from build123d import *

# Parameters (mm, degrees)
CUT_EXTRUDE1_DEPTH = 16.684387141
CIRPATTERN1_COUNT  = 6


with BuildPart() as part:
    # Sketch1 → Revolve1 (revolve)
    with BuildSketch(Plane.XY, mode=Mode.PRIVATE) as revolve1_sk:
        with BuildLine():
            Line((-5, 9), (-1.125, 9))
            Line((-1.125, 9), (-1.125, 4))
            Line((-1.125, 4), (0, 4))
            Line((0, 4), (0, -5))
            ThreePointArc((0, -5), (-3.535533906, -3.535533906), (-5, 0))
            Line((-5, 0), (-5, 9))
        make_face()
    revolve(revolve1_sk.sketch.rotate(Axis((0, 0, 0), (0, 1, 0)), 270), axis=Axis((0, 0, 0), (0, 1, 0)))

    # Sketch2 → Cut-Extrude1 (cut, through all)
    with BuildSketch(Plane(origin=(0, 9, 0), x_dir=(1, 0, 0), z_dir=(0, 1, 0))):
        with BuildLine():
            Line((-4.94979148, -0.706798632), (-3.36819132, 0))
            ThreePointArc((-3.36819132, 0), (-3.260778077, 0.247971643), (-3.498444432, 0.376588299))
            Line((-3.498444432, 0.376588299), (-5, 0))
            ThreePointArc((-5, 0), (-4.987432075, -0.354289854), (-4.94979148, -0.706798632))
        make_face()
    cut_extrude1 = extrude(amount=-CUT_EXTRUDE1_DEPTH, mode=Mode.SUBTRACT)

    # CirPattern1: Cut-Extrude1 ×6 about axis
    cirpattern1_axis = Axis((0, 0, 0), (0, 1, 0))
    for i in range(1, CIRPATTERN1_COUNT):
        add(cut_extrude1.rotate(cirpattern1_axis, i * 360 / CIRPATTERN1_COUNT), mode=Mode.SUBTRACT)


solid = part.part
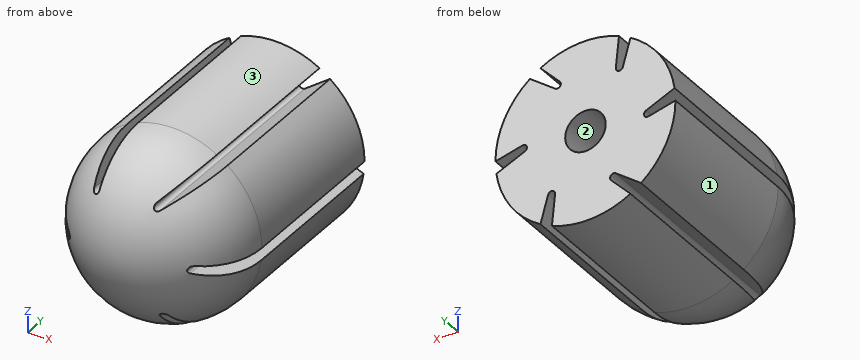
Check sheet for the modelled part. Datum: model origin and axes. Units: mm. Face numbers are marked on the shaded views. Coordinates: 2 decimals unless noted, no trailing zeros. Loops run counter-clockwise (first coordinate to the right, second up) from the corner with the lowest first, then second, coordinate; pieces in that order, holes last. Notation, with made-up numbers: (80, 30.25) -> (127, 30.25) arc R6 cw to (127, 40.25) -> close; hole circle Ø4 at (20.5, -37.5). An arc over 180 degrees is marked (long way). Answer in a Markdown table with one row per item.
1. Material ranges on line 1 along X through (y, z) = (8, -3); line 2 along X through (y, z) = (2.75, 3); line 3 along Z through (x, y) = (-3.5, 0.75), recorded low to high. Write a range as [from, to].
Check values:
| item | result |
|---|---|
| line 1 | x = [-4, -1.8], [-1.38, 1.69], [2.12, 4] |
| line 2 | x = [-4, -2.12], [-1.69, 1.38], [1.8, 4] |
| line 3 | z = [-3.57, -0.38], [0.06, 3.57] |
2. Sectioned sample at C-C, the plane y = 2. Record the boundary of the cut face in (x, z), then the cut area to 3 significant figures.
Check values:
| item | result |
|---|---|
| outline | (-5, 0) arc R5 ccw to (-3.09, -3.93) -> (-1.68, -2.92) arc R0.2 cw to (-1.42, -3.22) -> (-2.5, -4.33) arc R5 ccw to (1.86, -4.64) -> (1.68, -2.92) arc R0.2 cw to (2.08, -2.84) -> (2.5, -4.33) arc R5 ccw to (4.95, -0.71) -> (3.37, 0) arc R0.2 cw to (3.5, 0.38) -> (5, 0) arc R5 ccw to (3.09, 3.93) -> (1.68, 2.92) arc R0.2 cw to (1.42, 3.22) -> (2.5, 4.33) arc R5 ccw to (-1.86, 4.64) -> (-1.68, 2.92) arc R0.2 cw to (-2.08, 2.84) -> (-2.5, 4.33) arc R5 ccw to (-4.95, 0.71) -> (-3.37, 0) arc R0.2 cw to (-3.5, -0.38) -> close |
| area | 72.9 mm2 |
3. Release check for a two-part mould opening along Z. For the marked faces 1, 2 and 3 record: released by +Z, released by -Z, zero draft, split by the parting line, or undercut.
Check values:
| item | result |
|---|---|
| face 1 | released by -Z |
| face 2 | undercut |
| face 3 | released by +Z |
4. Sectioned sample at A-A, the plane y = 6.5. Record the boundary of the cut face in (x, z) (3 decimals).
Check values:
| item | result |
|---|---|
| outline | (-5, 0) arc R5 ccw to (-3.087, -3.933) -> (-1.684, -2.917) arc R0.2 cw to (-1.423, -3.218) -> (-2.5, -4.33) arc R5 ccw to (1.863, -4.64) -> (1.684, -2.917) arc R0.2 cw to (2.075, -2.841) -> (2.5, -4.33) arc R5 ccw to (4.95, -0.707) -> (3.368, 0) arc R0.2 cw to (3.498, 0.377) -> (5, 0) arc R5 ccw to (3.087, 3.933) -> (1.684, 2.917) arc R0.2 cw to (1.423, 3.218) -> (2.5, 4.33) arc R5 ccw to (-1.863, 4.64) -> (-1.684, 2.917) arc R0.2 cw to (-2.075, 2.841) -> (-2.5, 4.33) arc R5 ccw to (-4.95, 0.707) -> (-3.368, 0) arc R0.2 cw to (-3.498, -0.377) -> close; hole circle Ø2.25 at (0, 0) |
5. Sectioned sample at D-D, the plane x = -4.5. Record the boundary of the cut face in (y, z), then the cut area to 3 significant figures.
Check values:
| item | result |
|---|---|
| outline | (-2.18, -0.13) arc R2.18 ccw to (0, -2.18) -> (9, -2.18) -> (9, -0.13) -> close; (-2.12, 0.51) -> (9, 0.51) -> (9, 2.18) -> (0, 2.18) arc R2.18 ccw to start |
| area | 39.6 mm2 |
6. Go/stop test with flat-tipped pins: pin 1 (2.5 mm diameter, centred on x = -0.5, z = -0.5, fed in from +Y); pin 2 (1.5 mm diameter, centred on x = -1.5, y = -2, fed in from +Z); pin 3 (2 mm diameter, centred on x = 0, z = 0, fed in from +Y); pin 4 (6 mm diameter, centred on y = -3, z = -3.5, fed in from +X). Record where each tip stops, or that it passes through.
Check values:
| item | result |
|---|---|
| pin 1 | stops at y = 9 |
| pin 2 | stops at z = 4.68 |
| pin 3 | stops at y = 4 |
| pin 4 | stops at x = 4.73 |
7. Sectioned sample at B-B, the plane x = 0. Record the boundary of the cut face in (y, z) (3 decimals), then the cut area to 3 significant figures.
Check values:
| item | result |
|---|---|
| outline | (0, -5) -> (9, -5) -> (9, -1.125) -> (4, -1.125) -> (4, 1.125) -> (9, 1.125) -> (9, 5) -> (0, 5) arc R5 ccw to start |
| area | 118 mm2 |
